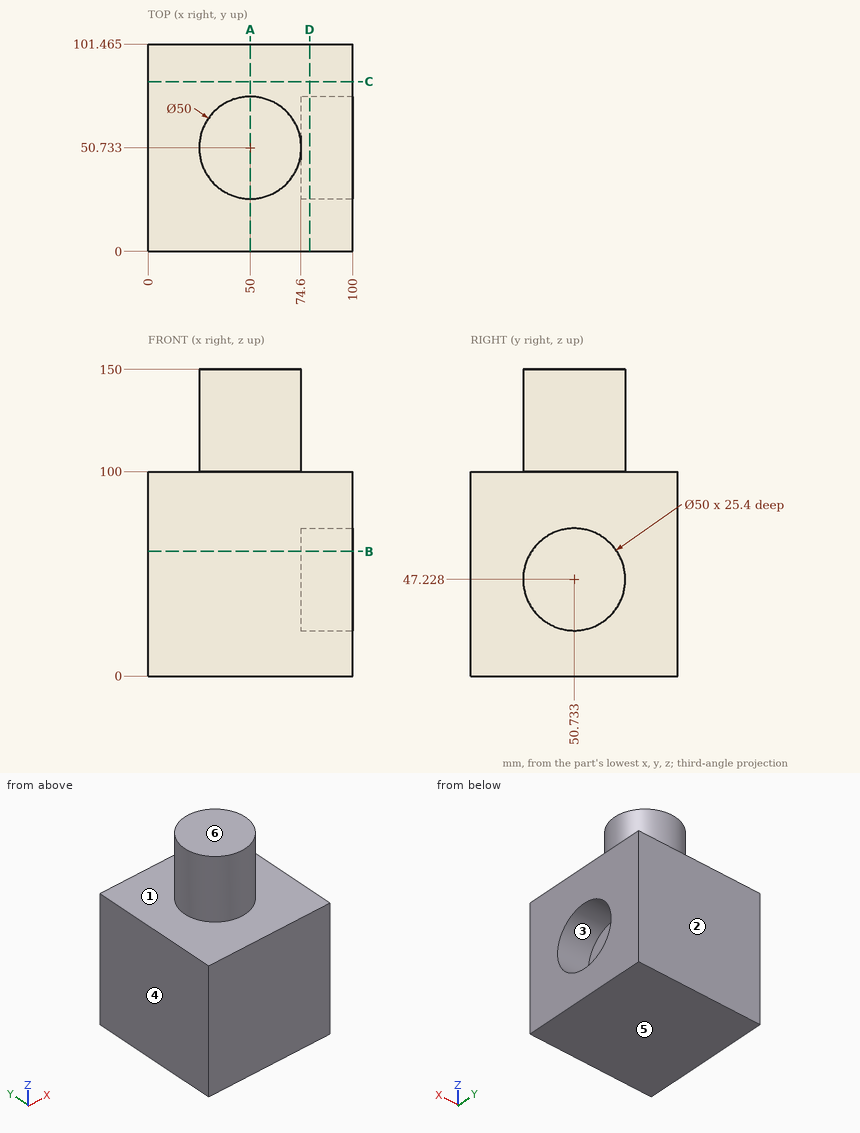
Part print with two shaded views. Sizes in mm from the minimum x, y, z corner. A direction names the side the tool comes from. Give positions to 0.01 mm unless a question says otherwise; leave off trailing zeros. Write each loop counter-clockwise with the first axis right and the second up, starting at its lowest first coordinate (ties: lowest second). Pieces come first, ordered by that corner, then holes.
1) Pin check, flat tip, straight feed: pin 1 (12 mm diameter, centred on x = 16, y = 90, fed in from +Z). Stop position of the tip, or through.
Resolved:
pin 1: stops at z = 100
2) Two-plate mould, pull along Z, no slides. Class the marked faces 3, 4, 5 and 6: released by +Z, released by -Z, zero draft, split by the parting line, or undercut.
Resolved:
face 3: undercut
face 4: zero draft
face 5: released by -Z
face 6: released by +Z
3) Cut at D-D on x = 79. Write the cut outline in (y, z) (1 decimal).
Resolved:
outline: (0, 0) - (101.5, 0) - (101.5, 100) - (0, 100) - close; hole circle Ø50 at (50.7, 47.2)
4) Cut at B-B on z = 61. Write the cut outline in (x, y) (1 decimal).
Resolved:
outline: (0, 0) - (100, 0) - (100, 29.9) - (74.6, 29.9) - (74.6, 71.6) - (100, 71.6) - (100, 101.5) - (0, 101.5) - close
5) Cut at A-A on x = 50. Write the cut outline in (y, z) (1 decimal), then the cut area to 3 significant figures.
Resolved:
outline: (0, 0) - (101.5, 0) - (101.5, 100) - (75.7, 100) - (75.7, 150) - (25.7, 150) - (25.7, 100) - (0, 100) - close
area: 12,600 mm2
6) Probe L1, parallel to X at y = 47, z = 45; L2, parallel to Z at x = 31, y = 86.5; L3, parallel to Y at x = 81, z = 67 (1 decimal). List the from-to ranges inside material, lowest first.
Resolved:
L1: x = 0 to 74.6
L2: z = 0 to 100
L3: y = 0 to 35.4, 66 to 101.5
7) Which spindle directions (+Z, -Z, +X, -X, +Y, -Y) get a long thin tool onto all of the face, cutting with end or side? Do the marked faces 1 and 2. Say none if no direction does.
Resolved:
face 1: +Z
face 2: +Z, -Z, +X, -X, +Y
8) Cut at C-C on y = 83. Write the cut outline in (x, z), then the cut area to 3 significant figures.
Resolved:
outline: (0, 0) - (100, 0) - (100, 100) - (0, 100) - close
area: 10,000 mm2
